Input: dimensioned drawing with shaded views. Units: mm. Origin: part minimum x, y, z. Round coordinates to 2 decimals unless told otherwise and drop trailing zeros. Order: outer loops, then holes, each group sorted by start corner. A loop starts at its lowest first (then second) coordinate and runs counter-clockwise, first axis right, second up.
Item 1: Line query: L1, parallel to Z at x = 19, y = 0.7 (1 decimal); L2, parallel to X at y = 1.1, z = 4; L3, parallel to X at y = 0.65, z = 14.5. Output: solid intervals per line, ascending.
Item 2: First-contact query: pin 1 (1.5 mm diameter, centred on x = 19.05, z = 60.706, fed in from -Y). Flat tip, straight axial feed; report the tip coordinate or a pass-through.
Item 3: Cut plane A-A on x = 19.05. Output: boundary loops of the cut face in (y, z).
Item 4: Cut plane B-B on y = 0.8. Output: boundary loops of the cut face in (x, z) (3 decimals).
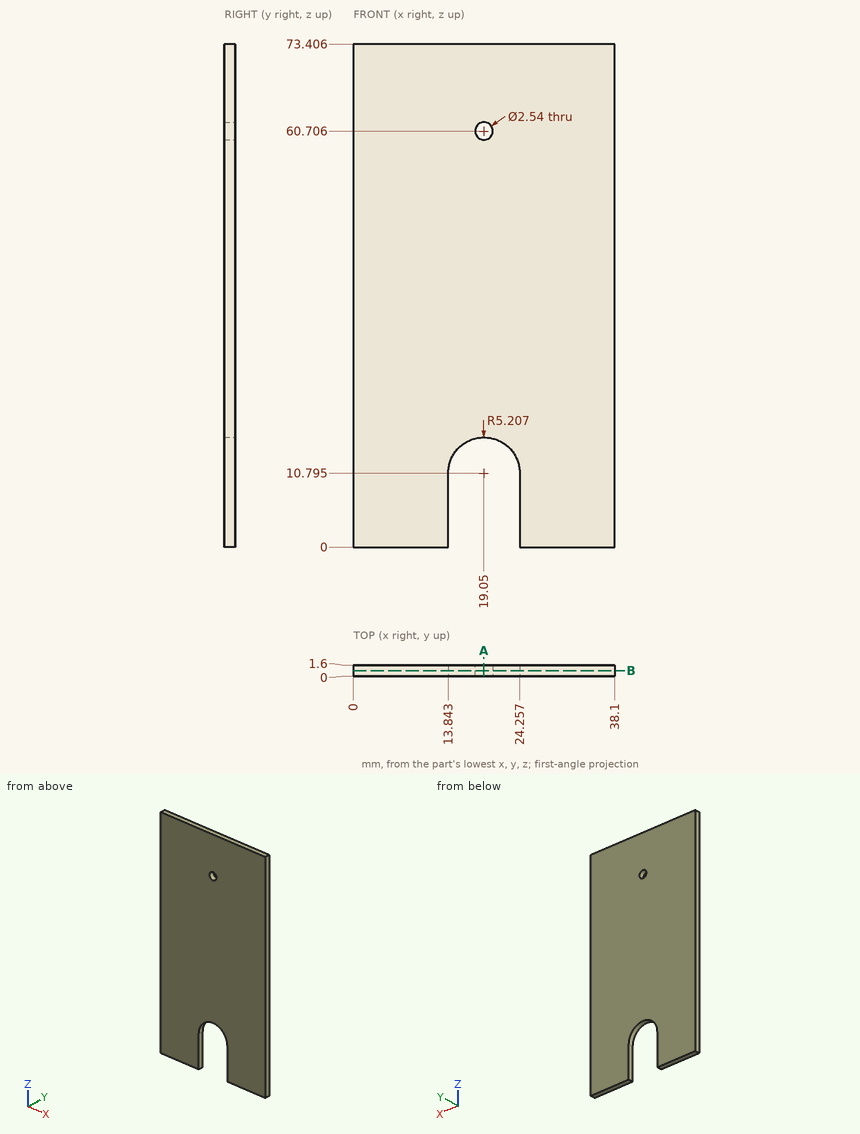
From the geometry:
1. L1: z = 16 to 59.4, 62 to 73.4
1. L2: x = 0 to 13.84, 24.26 to 38.1
1. L3: x = 0 to 15.39, 22.71 to 38.1
2. pin 1: passes through
3. outline: (0, 16) - (1.6, 16) - (1.6, 59.44) - (0, 59.44) - close; (0, 61.98) - (1.6, 61.98) - (1.6, 73.41) - (0, 73.41) - close
4. outline: (0, 0) - (13.843, 0) - (13.843, 10.795) arc R5.207 cw to (24.257, 10.795) - (24.257, 0) - (38.1, 0) - (38.1, 73.406) - (0, 73.406) - close; hole circle Ø2.54 at (19.05, 60.706)
